Can you work these out from the model? Positions are in its coordinate system, mm. A direction names the side the tool comes from. Give positions to 0.01 mm unless a question says otherwise; leave off trailing zeros. Loops run counter-clockwise (first coordinate to the right, second up) from the corner with the lowest first, then second, coordinate; pieces in that order, holes last. Notation, with made-up numbers: M 26.25,16 L 76.25,16 A32 ccw 76.25,47 Z; hole C 53,38 d4. An arc over 180 degrees is marked long. Put each result on its own line as item: value. Start each with the question number.
1) Please list where these lines run through material, in increasing order: line 1 along Y through (x, z) = (-5.5, -12) (3 decimals); line 2 along Y through (x, z) = (12.5, 3.5); line 3 along X through (y, z) = (5, -5). Write a range as from..to.
2) For P1, Ø3.5, axis at x = -0.5, z = -14, coming from the +Y side; P2, Ø2, axis at x = 17.5, z = -1.5, coming from the +Y side; P3, Ø4, axis at x = 26.5, y = 12, coming from the -Z side, each with a flat end and sliding along its axis, tell me the tip position at first contact or that it passes through.
3) For faces 1 (the cylindrical face through (19, 16.3, 2.5)), 2 (the cylindrical face through (7.64, -3.1, -12.62)), 3 (the cylindrical face through (-7.6, -3.14, -12.62)), 4 (the flat face through (29, 13, 0)), 5 (the flat face through (0, -16, 0)), which set-ups out of +Z, -Z, +X, -X, +Y, -Y let a thin tool reach every point of the face, with its end or its side?
4) If we mould it in two halves opening along Y, with no side actions, what happens to faces 6 (the flat face through (0, -4, -7)), 7 (the flat face through (-5, 7, -4)), 8 (the flat face through (-3, -17, 5)), 9 (the cylindrical face through (5.83, 5.66, -12.38))? For each: +Y half, -Y half, draft (parallel to the pull), parting line (faces both ways), or undercut.
5) Imagine slicing it at A-A (y = 16.25). Write out the boundary of the cut face in (x, z).
6) Imagine slicing it at B-B (x = 30). Write out the boundary of the cut face in (y, z), then the cut area to 3 significant figures.
7) Imagine slicing it at C-C (z = -16). Write out the boundary of the cut face in (x, y) (3 decimals), then the cut area to 3 significant figures.
from build123d import *

# Parameters (mm, degrees)
BOSS_EXTRUDE1_DEPTH = 5
BOSS_EXTRUDE2_START = 4
BOSS_EXTRUDE2_DEPTH = 4
FILLET1_R           = 4
SKETCH5_W           = 17
SKETCH5_H           = 4
BOSS_EXTRUDE3_DEPTH = 6.25
SKETCH8_W           = 17
SKETCH8_H           = 14.25
BOSS_EXTRUDE4_DEPTH = 17
SKETCH6_R           = 1.5
CUT_EXTRUDE1_DEPTH  = 45.484596337
FILLET3_R           = 3


with BuildPart() as part:
    # Sketch3 → Boss-Extrude1 (new body)
    with BuildSketch(Plane.XY):
        with BuildLine():
            Line((-20, -17.25), (20, -17.25))
            ThreePointArc((20, -17.25), (37.25, 0), (20, 17.25))
            ThreePointArc((20, 17.25), (19, 16.25), (20, 15.25))
            ThreePointArc((20, 15.25), (35.25, 0), (20, -15.25))
            Line((20, -15.25), (-20, -15.25))
            ThreePointArc((-20, -15.25), (-35.25, 0), (-20, 15.25))
            ThreePointArc((-20, 15.25), (-19, 16.25), (-20, 17.25))
            ThreePointArc((-20, 17.25), (-37.25, 0), (-20, -17.25))
        make_face()
    extrude(amount=BOSS_EXTRUDE1_DEPTH)

    # Sketch4 → Boss-Extrude2 (add)
    with BuildSketch(Plane(origin=(0, 0, 0), x_dir=(-1, 0, 0), z_dir=(0, 0, -1)).offset(BOSS_EXTRUDE2_START)):
        with BuildLine():
            Line((-36.779824195, 4), (36.779824195, 4))
            ThreePointArc((36.779824195, 4), (37.313761542, 0), (36.779824195, -4))
            Line((36.779824195, -4), (-36.779824195, -4))
            ThreePointArc((-36.779824195, -4), (-37.25, 0), (-36.779824195, 4))
        make_face()
    extrude(amount=-BOSS_EXTRUDE2_DEPTH)

    # Fillet1
    fillet1_edges = [part.edges().sort_by_distance(p)[0] for p in [
        (-37.313761542, 0, -4),
        (37.25, 0, -4),
    ]]
    fillet(fillet1_edges, radius=FILLET1_R - 0.0001)  # a hair under: the kernel refuses the full size

    # Sketch5 → Boss-Extrude3 (add)
    with BuildSketch(Plane(origin=(0, 4, 0), x_dir=(1, 0, 0), z_dir=(0, 1, 0))):
        with Locations((0, 2)):
            Rectangle(SKETCH5_W, SKETCH5_H)
    extrude(amount=BOSS_EXTRUDE3_DEPTH)

    # Sketch8 → Boss-Extrude4 (add)
    with BuildSketch(Plane(origin=(0, 0, -4), x_dir=(-1, 0, 0), z_dir=(0, 0, -1))):
        with Locations((0, 3.125)):
            Rectangle(SKETCH8_W, SKETCH8_H)
    extrude(amount=BOSS_EXTRUDE4_DEPTH)

    # Sketch6 → Cut-Extrude1 (cut, through all)
    with BuildSketch(Plane(origin=(0, 0, -4), x_dir=(-1, 0, 0), z_dir=(0, 0, -1))):
        with Locations((-5.5, 7.125)):
            Circle(SKETCH6_R)
        with Locations((5.5, 7.125)):
            Circle(SKETCH6_R)
    extrude(amount=CUT_EXTRUDE1_DEPTH, mode=Mode.SUBTRACT)

    # Fillet3
    fillet3_edges = [part.edges().sort_by_distance(p)[0] for p in [
        (-8.5, 10.25, -10.5),
        (8.5, 10.25, -10.5),
        (8.5, -4, -12.5),
        (-8.5, -4, -12.5),
    ]]
    fillet(fillet3_edges, radius=FILLET3_R)


solid = part.part
Recorded:
1. line 1: -4..5.625, 8.625..10.25
1. line 2: -17.25..-15.25
1. line 3: -8.5..8.5
2. P1: y = 10.25
2. P2: y = 4
2. P3: z = 0
3. face 1: +Z, -Z
3. face 2: -Z, +X, -Y
3. face 3: -Z, -X, -Y
3. face 4: -Z, +X, +Y
3. face 5: -Z, +X, -X, -Y
4. face 6: -Y half
4. face 7: undercut
4. face 8: draft
4. face 9: undercut
5. outline: M -25.79,0 L -19,0 L -19,5 L -25.79,5 Z; M 19,0 L 25.79,0 L 25.79,5 L 19,5 Z
6. outline: M -14.06,0 L -11.51,0 L -11.51,5 L -14.06,5 Z; M -4,-4 L 4,-4 L 4,0 L -4,0 Z; M 11.51,0 L 14.06,0 L 14.06,5 L 11.51,5 Z
6. area: 57.4 mm²
7. outline: M -8.5,-1 A3 ccw -5.5,-4 L 5.5,-4 A3 ccw 8.5,-1 L 8.5,7.25 A3 ccw 5.5,10.25 L -5.5,10.25 A3 ccw -8.5,7.25 Z; hole C -5.5,7.125 d3; hole C 5.5,7.125 d3
7. area: 220 mm²
